For this review, take the finished solid that the model builds, in its own axes (mm). Give positions to 0.01 mm unless a question says otherwise; leave off trailing zeros. Write each loop counter-clockwise with the first axis right and the second up, starting at its lowest first coordinate (ties: lowest second). Pieces come first, ordered by that corner, then holes. Notation, with made-up numbers: (-21.5, 5) -> (23.5, 5) arc R17 cw to (23.5, 28) -> close; hole circle Ø1 at (-7, 15.5). An arc over 180 degrees is marked (long way). Return JSON: item names as keys, results as strings.
from build123d import *

# Parameters (mm, degrees)
F0_R          = 10
F1_DEPTH      = 58
F2_R          = 8
F3_DEPTH      = 60
F4_R          = 2.5
F5_DEPTH      = 25
F5_DEPTH_BACK = 25


with BuildPart() as f1:
    # F0 (on Front) → F1 (new body)
    with BuildSketch(Plane.XZ):
        Circle(F0_R)
    extrude(amount=F1_DEPTH)

    # F2 (on face) → F3 (cut)
    with BuildSketch(Plane.XZ.offset(58)):
        Circle(F2_R)
    extrude(amount=-F3_DEPTH, mode=Mode.SUBTRACT)

    # F4 (on Top) → F5 (cut, two sides)
    with BuildSketch(Plane.XY) as f5_sk:
        with Locations((0, -6.5)):
            Circle(F4_R)
    extrude(amount=-F5_DEPTH, mode=Mode.SUBTRACT)
    extrude(f5_sk.sketch, amount=F5_DEPTH_BACK, mode=Mode.SUBTRACT)


solid = f1.part
1. For pin 1 (6 mm diameter, centred on x = -6.5, y = -14, fed in from +Z); pin 2 (5 mm diameter, centred on y = -12, z = 6, fed in from +X); pin 3 (1.5 mm diameter, centred on y = -52, z = -2.5, fed in from +X), all flat-tipped, find the tip position at first contact; note any pin that passes through.
Results found:
{"pin 1": "stops at z = 9.37", "pin 2": "stops at x = 9.37", "pin 3": "stops at x = 9.85"}
2. The part is to be moulded in two halves that separate along X. For faces 1 (the flat face through (0, 0, 8.2)), 2 (the cylindrical face through (-2.17, -28.59, -9.76)), 3 (the cylindrical face through (-1.73, -29.41, -7.81)), say which applies: +X half, -X half, draft (parallel to the pull), parting line (faces both ways), or undercut.
Results found:
{"face 1": "draft", "face 2": "parting line", "face 3": "undercut"}
3. Add section B-B, the plane x = -3.25. State the section outline as (y, z) points.
Results found:
{"outline": "(-58, -9.46) -> (0, -9.46) -> (0, -7.31) -> (-58, -7.31) -> close; (-58, 7.31) -> (0, 7.31) -> (0, 9.46) -> (-58, 9.46) -> close"}
4. To check wall thickness, follow probe 1 along X at (y, z) = (-10.5, -0.25); probe 2 along Z at (x, y) = (-3, -40.5). State the ranges of each line that lie inside material, in increasing order.
Results found:
{"probe 1": "x = -10 to -8, 8 to 10", "probe 2": "z = -9.54 to -7.42, 7.42 to 9.54"}
5. Add section C-C, the plane y = -38.5. State the section outline as (x, z) points.
Results found:
{"outline": "circle Ø20 at (0, 0); hole circle Ø16 at (0, 0)"}
6. Add section A-A, the plane z = 0. State the section outline as (x, y) points, plus the area to 3 significant figures.
Results found:
{"outline": "(-10, -58) -> (-8, -58) -> (-8, 0) -> (-10, 0) -> close; (8, -58) -> (10, -58) -> (10, 0) -> (8, 0) -> close", "area": "232 mm²"}
